Part model, mm, in its own coordinate system. Face numbers are marked on the shaded views. A direction names the side the tool comes from. Coordinates: 2 decimals unless noted, no trailing zeros. Loops run counter-clockwise (first coordinate to the right, second up) from the corner with the lowest first, then second, coordinate; pieces in that order, holes last. Notation, with made-up numbers: M 48,-4 L 88,-4 A30 ccw 88,34 Z; hole C -28.75,46 d9. An arc over 180 degrees is marked long. Use a Markdown table: item, result. Add a question column.
1) Band-saw the part on C-C (z = 11.5). List the corners of the cut face in (x, y), plus the area to 3 significant figures.
2) Wall check: probe 1 along X at (y, z) = (0, -2.5); probe 2 along Z at (x, y) = (2, 11); probe 3 along Z at (x, y) = (10, 5.5). Give the ranges that are in metal, low to high. Write a range as from..to.
3) Tool access for the marked faces 1, 2 and 3: list every direction of +Z, -Z, +X, -X, +Y, -Y with a clear straight run to the whole face (end or side of a thin tool).
4) Pin check, flat tips, straight feed: pin 1 Ø8 at (y, z) = (0.5, -36.5) entering from -X; pin 2 Ø2.5 at (x, y) = (-14.5, 0) entering from +Z; pin 3 Ø3 at (x, z) = (-8, -48.5) entering from +Y. Stop position of each tip, or through.
5) Band-saw the part on D-D (z = -6). List the corners of the cut face in (x, y).
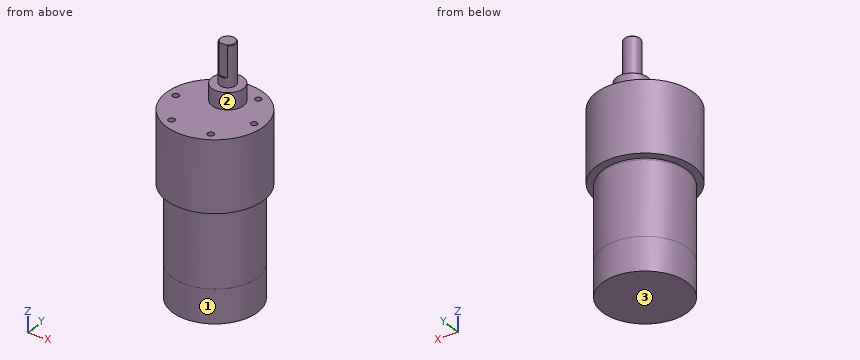
Autodesk Inventor part; units mm, degrees
ref_plane "YZ Plane" through (0, 0, 0) normal (1, 0, 0) x (0, 1, 0)
ref_plane "XZ Plane" through (0, 0, 0) normal (0, 1, 0) x (-1, 0, 0)
ref_plane "XY Plane" through (0, 0, 0) normal (0, 0, 1) x (1, 0, 0)
sketch "Sketch2" plane through (0, 0, 0) normal (1, 0, 0) x (0, 1, 0)
  line L0 (0, 0) -> (0, -90.5559) construction
  line L1 (0, 0) -> (18.5, 0)
  line L2 (18.5, 0) -> (18.5, -27)
  line L3 (18.5, -27) -> (0, -27)
  line L4 (0, -27) -> (0, 0)
  line L5 (0, -27) -> (16.15, -27)
  line L6 (16.15, -28) -> (16.15, -56)
  line L7 (16.15, -56) -> (0, -56)
  line L8 (0, -56) -> (0, -27)
  line L9 (0, -56) -> (16.16, -56)
  line L10 (16.16, -56) -> (16.16, -68.7)
  line L11 (16.16, -68.7) -> (0, -68.7)
  line L12 (0, -68.7) -> (0, -56)
  arc A0 (16.15, -28) -> (15.15, -27) centre (15.15, -28) ccw
  line L13 (16.15, -28) -> (15.15, -28) construction
  line L14 (15.15, -27) -> (15.15, -28) construction
  dimension "d1" = 27
  dimension "d3" = 41.7
  dimension "d4" = 37
  dimension "d5" = 0.01
  dimension "d6" = 2.35
  dimension "d7" = 29
  dimension "d8" = 1
  dimension "d9" = 90
revolve "Revolution1" add sketch "Sketch2" angle 360 about axis through (0, 0, 0) along (0, 0, -1)
sketch "Sketch4" plane through (0, 0, 0) normal (1, 0, 0) x (0, 1, 0)
  line L0 (7, 0) -> (7, 36.4313)
  line L1 (7, 0) -> (0, 0)
  line L2 (-18.5, 0) -> (18.5, 0)
  line L3 (7, 0) -> (13, 0)
  line L4 (13, 0) -> (13, 6.3)
  line L5 (13, 6.3) -> (7, 6.3)
  line L6 (7, 6.3) -> (7, 0)
  line L7 (7, 6.3) -> (10, 6.3)
  line L8 (10, 6.3) -> (10, 21.8)
  line L9 (10, 21.8) -> (7, 21.8)
  line L10 (7, 21.8) -> (7, 6.3)
  dimension "d12" = 7
  dimension "d13" = 6.3
  dimension "d14" = 12
  dimension "d15" = 15.5
  dimension "d16" = 6
revolve "Revolution2" add sketch "Sketch4" angle 360 about axis through (0, 7, 0) along (0, 0, 1)
chamfer "Chamfer1" distance 0.25 angle 45 1 edges at (0, 4, 21.8)
sketch "Sketch5" plane through (0, 7, 21.8) normal (0, 0, 1) x (1, 0, 0)
  circle A0 centre (0, 0) radius 3
  line L0 (-1.6583, -2.5) -> (1.6583, -2.5)
  point P0 (0, -7)
  point P1 (0, 3)
  dimension "d18" = 5.5
extrude "Extrusion1" cut sketch "Sketch5" against normal blind 12 contours L0 A0 picked at (-0.3442, -2.6056)
sketch "Sketch6" plane through (0, 0, 0) normal (0, 0, 1) x (1, 0, 0)
  point P0 (0, 0)
  point P1 (-15, 0)
  dimension "d24" = 15
hole "Hole1" at (-15, 0, 0) direction (0, 0, -1) diameter 2.459 depth 3.5
pattern_circular "Circular Pattern1" count 6 over 360 about axis through (0, 0, -13.5) along (0, 0, -1) of "Hole1"
equation "\"BendRadius\" = Thickness"
equation "\"BendReliefWidth\" = Thickness"
equation "\"BendReliefDepth\" = 0.5 * Thickness"
equation "\"CornerReliefSize\" = 4 * Thickness"
equation "\"MinimumRemnant\" = 2 * Thickness"
equation "\"TransitionRadius\" = BendRadius"
equation "\"JacobiRadiusSize\" = BendRadius"
equation "\"GapSize\" = Thickness"
properties part number "Vince-Motor"
Entries:
| question | item | result |
|---|---|---|
| 1 | outline | M -1.66,4.5 L 1.66,4.5 A3 ccw long Z |
| 1 | area | 27.1 mm2 |
| 2 | probe 1 | -18.5..-16.23, -13.77..13.77, 16.23..18.5 |
| 2 | probe 2 | -68.7..6.3 |
| 2 | probe 3 | -68.7..0 |
| 3 | face 1 | -Z |
| 3 | face 2 | +Z |
| 3 | face 3 | -Z, +X, -X, +Y, -Y |
| 4 | pin 1 | x = -16.15 |
| 4 | pin 2 | z = 0 |
| 4 | pin 3 | y = 14.78 |
| 5 | outline | C 0,0 d37 |
